Can you work these out from the model? Positions are in its coordinate system, mm. Give positions to 0.01 mm unless a question says otherwise; leave off trailing zeros. Loops run counter-clockwise (first coordinate to the right, second up) from the corner with the lowest first, then second, coordinate; pieces in that order, holes last. Notation, with made-up numbers: M 11.5,53 L 62.5,53 A7 ccw 62.5,58 Z; hole C -3,3 d8. An arc over 180 degrees is marked long. One line per item, written item: value. Start each with the question number.
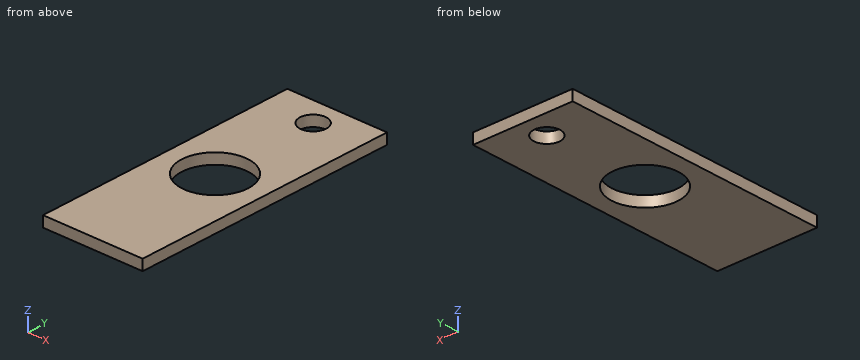
from build123d import *

# Parameters (mm, degrees)
SKETCH1_W                    = 19.05
SKETCH1_H                    = 50.8
SKETCH1_R                    = 6.35
BOSS_EXTRUDE1_DEPTH          = 2
F_5_0_5_DIAMETER_HOLE1_D     = 5
F_5_0_5_DIAMETER_HOLE1_DEPTH = 5
F_5_0_5_DIAMETER_HOLE1_TIP   = 1.502151548


with BuildPart() as part:
    # Sketch1 → Boss-Extrude1 (new body)
    with BuildSketch(Plane.XY):
        Rectangle(SKETCH1_W, SKETCH1_H)
        Circle(SKETCH1_R, mode=Mode.SUBTRACT)
    extrude(amount=BOSS_EXTRUDE1_DEPTH)

    # Ø5.0 (5) Diameter Hole1
    with Locations(Plane(origin=(0, 0, 0), x_dir=(-1, 0, 0), z_dir=(0, 0, -1))):
        with Locations((0, 20.4)):
            Hole(F_5_0_5_DIAMETER_HOLE1_D / 2, depth=F_5_0_5_DIAMETER_HOLE1_DEPTH)
            with Locations((0, 0, -(F_5_0_5_DIAMETER_HOLE1_DEPTH + F_5_0_5_DIAMETER_HOLE1_TIP / 2))):  # 118° drill point
                Cone(0, F_5_0_5_DIAMETER_HOLE1_D / 2, F_5_0_5_DIAMETER_HOLE1_TIP, mode=Mode.SUBTRACT)


solid = part.part
Q1. For P1, Ø10, axis at x = 0, y = 0, coming from the -Z side; P2, Ø6, axis at x = 0, y = 20.4, coming from the +Z side, each with a flat end and sliding along its axis, tell me the tip position at first contact or that it passes through.
Q2. I need wall thicknesses on line 1 along Y through (x, z) = (0, 1.5); line 2 along Y through (x, z) = (-0.5, 0.4); line 3 along X through (y, z) = (-5, 1) (3 decimals). Which ranges of each line are inside material? Lowest first, please.
Q3. If we section it at A-A, the plane y = 20.4: Write out the boundary of the cut face in (x, z) (3 decimals).
Q4. If we section it at B-B, the plane x = 0: Write out the boundary of the cut face in (y, z), plus the area to 3 significant figures.
Q5. If we section it at D-D, the plane x = 3.75: Write out the boundary of the cut face in (y, z), plus the area to 3 significant figures.
Q6. If we section it at C-C, the plane z = 1.1: Write out the boundary of the cut face in (x, y) (3 decimals), plus the area to 3 significant figures.
Response:
1. P1: through
1. P2: z = 2
2. line 1: -25.4 to -6.35, 6.35 to 17.9, 22.9 to 25.4
2. line 2: -25.4 to -6.33, 6.33 to 17.95, 22.85 to 25.4
2. line 3: -9.525 to -3.914, 3.914 to 9.525
3. outline: M -9.525,0 L -2.5,0 L -2.5,2 L -9.525,2 Z; M 2.5,0 L 9.525,0 L 9.525,2 L 2.5,2 Z
4. outline: M -25.4,0 L -6.35,0 L -6.35,2 L -25.4,2 Z; M 6.35,0 L 17.9,0 L 17.9,2 L 6.35,2 Z; M 22.9,0 L 25.4,0 L 25.4,2 L 22.9,2 Z
4. area: 66.2 mm^2
5. outline: M -25.4,0 L -5.12,0 L -5.12,2 L -25.4,2 Z; M 5.12,0 L 25.4,0 L 25.4,2 L 5.12,2 Z
5. area: 81.1 mm^2
6. outline: M -9.525,-25.4 L 9.525,-25.4 L 9.525,25.4 L -9.525,25.4 Z; hole C 0,0 d12.7; hole C 0,20.4 d5
6. area: 821 mm^2
